from build123d import *

# Parameters (mm, degrees)
ESQUISSE1_W             = 180
ESQUISSE1_H             = 50
ESQUISSE1_R             = 3
BOSS_EXTRU_1_DEPTH      = 5
ESQUISSE2_W             = 75
ESQUISSE2_H             = 15
BOSS_EXTRU_2_DEPTH      = 75
ESQUISSE3_R             = 15
ENL_V_MAT_EXTRU_1_DEPTH = 15
ESQUISSE4_R             = 31
ENL_V_MAT_EXTRU_2_DEPTH = 10
CONG_1_R                = 20
CHANFREIN1_SIZE         = 15
CHANFREIN1_SIZE2        = 12.586494468
CONG_2_R                = 20
ESQUISSE5_W             = 10
ESQUISSE5_H             = 10
ENL_V_MAT_EXTRU_3_DEPTH = 5


with BuildPart() as part:
    # Esquisse1 → Boss.-Extru.1 (new body)
    with BuildSketch(Plane.XY):
        with Locations((5.796013405, 25)):
            Rectangle(ESQUISSE1_W, ESQUISSE1_H)
        with Locations((40.796013405, 6)):
            Circle(ESQUISSE1_R, mode=Mode.SUBTRACT)
        with Locations((-69.406004871, 22.939397164)):
            Circle(ESQUISSE1_R, mode=Mode.SUBTRACT)
        with Locations((-40.981469067, 6.77616521)):
            Circle(ESQUISSE1_R, mode=Mode.SUBTRACT)
        with Locations((-8.861542866, 12.901085106)):
            Circle(ESQUISSE1_R, mode=Mode.SUBTRACT)
        with Locations(Location((-29.203986595, 6, 0), (0, 0, 180))):
            Circle(ESQUISSE1_R, mode=Mode.SUBTRACT)
        with Locations(Location((80.99803168, 22.939397164, 0), (0, 0, 180))):
            Circle(ESQUISSE1_R, mode=Mode.SUBTRACT)
        with Locations(Location((52.573495876, 6.77616521, 0), (0, 0, 180))):
            Circle(ESQUISSE1_R, mode=Mode.SUBTRACT)
        with Locations(Location((20.453569676, 12.901085106, 0), (0, 0, 180))):
            Circle(ESQUISSE1_R, mode=Mode.SUBTRACT)
    extrude(amount=BOSS_EXTRU_1_DEPTH)

    # Esquisse2 → Boss.-Extru.2 (add)
    with BuildSketch(Plane.XY.offset(5)):
        with Locations((5.796013405, 42.5)):
            Rectangle(ESQUISSE2_W, ESQUISSE2_H)
    extrude(amount=BOSS_EXTRU_2_DEPTH)

    # Esquisse3 → Enlèv. mat.-Extru.1 (cut)
    with BuildSketch(Plane(origin=(0, 50, 0), x_dir=(1, 0, 0), z_dir=(0, 1, 0))):
        with Locations(Location((5.796013405, -42.5, 0), (0, 0, 270))):
            Circle(ESQUISSE3_R)
    extrude(amount=-ENL_V_MAT_EXTRU_1_DEPTH, mode=Mode.SUBTRACT)

    # Esquisse4 → Enlèv. mat.-Extru.2 (cut)
    with BuildSketch(Plane(origin=(0, 50, 0), x_dir=(1, 0, 0), z_dir=(0, 1, 0))):
        with Locations(Location((5.796013405, -42.5, 0), (0, 0, 270))):
            Circle(ESQUISSE4_R)
    extrude(amount=-ENL_V_MAT_EXTRU_2_DEPTH, mode=Mode.SUBTRACT)

    # Congé1
    cong_1_edges = [part.edges().sort_by_distance(p)[0] for p in [
        (43.296013405, 42.5, 80),
        (-31.703986595, 42.5, 80),
    ]]
    fillet(cong_1_edges, radius=CONG_1_R)

    # Chanfrein1
    chanfrein1_edges = [part.edges().sort_by_distance(p)[0] for p in [
        (5.796013405, 35, 5),
    ]]
    chanfrein1_side = [part.faces().sort_by_distance(p)[0] for p in [
        (5.796013405, 22.805952806, 5),
    ]]
    chamfer(chanfrein1_edges, length=CHANFREIN1_SIZE, length2=CHANFREIN1_SIZE2, reference=chanfrein1_side[0])

    # Congé2
    # the kernel refuses this fillet: 20 mm, written as the material it adds along each edge
    with BuildSketch(Plane(origin=(-31.703986595, -30, 5), x_dir=(0, 0, 1), z_dir=(0, 1, 0))) as cong_2_piece_1_section:
        with BuildLine():
            CenterArc((CONG_2_R, -CONG_2_R), CONG_2_R, 90, 90)
            Line((0, -CONG_2_R), (0, 0))
            Line((0, 0), (CONG_2_R, 0))
        make_face()
    cong_2_piece_1 = extrude(amount=80, mode=Mode.PRIVATE)
    cong_2_piece_1 = split(cong_2_piece_1, bisect_by=Plane(origin=(-37.472324852, 26.525505275, 10.475549069), z_dir=(0, 0.6427876096865406, -0.766044443118977)), keep=Keep.TOP, mode=Mode.PRIVATE)
    cong_2_piece_1 = split(cong_2_piece_1, bisect_by=Plane(origin=(-37.472324852, 35, 7.522714945), z_dir=(0, -1, 0)), keep=Keep.TOP, mode=Mode.PRIVATE)
    add(cong_2_piece_1)
    with BuildSketch(Plane(origin=(-31.703986595, -30, 5), x_dir=(0, 0, 1), z_dir=(0, 1, 0))) as cong_2_piece_2_section:
        with BuildLine():
            CenterArc((CONG_2_R, -CONG_2_R), CONG_2_R, 90, 90)
            Line((0, -CONG_2_R), (0, 0))
            Line((0, 0), (CONG_2_R, 0))
        make_face()
    cong_2_piece_2 = extrude(amount=80, mode=Mode.PRIVATE)
    cong_2_piece_2 = split(cong_2_piece_2, bisect_by=Plane(origin=(-31.680860217, 38.546515029, 20.562373921), z_dir=(0, -0.6427876096865406, 0.766044443118977)), keep=Keep.TOP, mode=Mode.PRIVATE)
    cong_2_piece_2 = split(cong_2_piece_2, bisect_by=Plane(origin=(-31.680860217, 35, 21.798113742), z_dir=(0, 1, 0)), keep=Keep.TOP, mode=Mode.PRIVATE)
    add(cong_2_piece_2)
    with BuildSketch(Plane(origin=(-31.703986595, -30, 5), x_dir=(0, 0, 1), z_dir=(0, 1, 0))) as cong_2_piece_3_section:
        with BuildLine():
            CenterArc((CONG_2_R, -CONG_2_R), CONG_2_R, 90, 90)
            Line((0, -CONG_2_R), (0, 0))
            Line((0, 0), (CONG_2_R, 0))
        make_face()
    cong_2_piece_3 = extrude(amount=80, mode=Mode.PRIVATE)
    cong_2_piece_3 = split(cong_2_piece_3, bisect_by=Plane(origin=(-36.294325359, 35.39038505, 17.914066419), z_dir=(0, 0.6427876096865406, -0.766044443118977)), keep=Keep.TOP, mode=Mode.PRIVATE)
    cong_2_piece_3 = split(cong_2_piece_3, bisect_by=Plane(origin=(-36.294325359, 35, 9.359564784), z_dir=(0, 1, 0)), keep=Keep.TOP, mode=Mode.PRIVATE)
    add(cong_2_piece_3)
    with BuildSketch(Plane(origin=(43.296013405, -30, 5), x_dir=(0, 0, 1), z_dir=(0, 1, 0))) as cong_2_piece_4_section:
        with BuildLine():
            CenterArc((CONG_2_R, CONG_2_R), CONG_2_R, 180, 90)
            Line((0, CONG_2_R), (0, 0))
            Line((0, 0), (CONG_2_R, 0))
        make_face()
    cong_2_piece_4 = extrude(amount=80, mode=Mode.PRIVATE)
    cong_2_piece_4 = split(cong_2_piece_4, bisect_by=Plane(origin=(49.064351662, 35, 7.522714945), z_dir=(0, -1, 0)), keep=Keep.TOP, mode=Mode.PRIVATE)
    cong_2_piece_4 = split(cong_2_piece_4, bisect_by=Plane(origin=(49.064351662, 26.525505275, 10.475549069), z_dir=(0, 0.6427876096865406, -0.766044443118977)), keep=Keep.TOP, mode=Mode.PRIVATE)
    add(cong_2_piece_4)
    with BuildSketch(Plane(origin=(43.296013405, -30, 5), x_dir=(0, 0, 1), z_dir=(0, 1, 0))) as cong_2_piece_5_section:
        with BuildLine():
            CenterArc((CONG_2_R, CONG_2_R), CONG_2_R, 180, 90)
            Line((0, CONG_2_R), (0, 0))
            Line((0, 0), (CONG_2_R, 0))
        make_face()
    cong_2_piece_5 = extrude(amount=80, mode=Mode.PRIVATE)
    cong_2_piece_5 = split(cong_2_piece_5, bisect_by=Plane(origin=(43.272887026, 35, 21.798113742), z_dir=(0, 1, 0)), keep=Keep.TOP, mode=Mode.PRIVATE)
    cong_2_piece_5 = split(cong_2_piece_5, bisect_by=Plane(origin=(43.272887026, 38.546515029, 20.562373921), z_dir=(0, -0.6427876096865406, 0.766044443118977)), keep=Keep.TOP, mode=Mode.PRIVATE)
    add(cong_2_piece_5)
    with BuildSketch(Plane(origin=(43.296013405, -30, 5), x_dir=(0, 0, 1), z_dir=(0, 1, 0))) as cong_2_piece_6_section:
        with BuildLine():
            CenterArc((CONG_2_R, CONG_2_R), CONG_2_R, 180, 90)
            Line((0, CONG_2_R), (0, 0))
            Line((0, 0), (CONG_2_R, 0))
        make_face()
    cong_2_piece_6 = extrude(amount=80, mode=Mode.PRIVATE)
    cong_2_piece_6 = split(cong_2_piece_6, bisect_by=Plane(origin=(47.886352168, 35, 9.359564784), z_dir=(0, 1, 0)), keep=Keep.TOP, mode=Mode.PRIVATE)
    cong_2_piece_6 = split(cong_2_piece_6, bisect_by=Plane(origin=(47.886352168, 35.39038505, 17.914066419), z_dir=(0, 0.6427876096865406, -0.766044443118977)), keep=Keep.TOP, mode=Mode.PRIVATE)
    add(cong_2_piece_6)

    # Esquisse5 → Enlèv. mat.-Extru.3 (cut)
    with BuildSketch(Plane.XY.offset(5)):
        with Locations((-79.203986595, 5)):
            Rectangle(ESQUISSE5_W, ESQUISSE5_H)
        with Locations((90.796013405, 5)):
            Rectangle(ESQUISSE5_W, ESQUISSE5_H)
    extrude(amount=-ENL_V_MAT_EXTRU_3_DEPTH, mode=Mode.SUBTRACT)


solid = part.part
Work out the finished part from the listing and answer in its coordinate system (mm). A direction names the side the tool comes from. Round coordinates to 2 decimals unless told otherwise and drop trailing zeros. Write each loop counter-clockwise with the first axis right and the second up, starting at its lowest first coordinate (ties: lowest second). Pieces come first, ordered by that corner, then holes. Notation, with made-up numbers: (77, 84.25) -> (126, 84.25) arc R22 cw to (126, 93.25) -> close; hole circle Ø3 at (-8.5, 55). An arc over 180 degrees is marked (long way). Write each question's results on one line, items separated by ' | '.
Item 1: Flat-ended cylindrical pins translate along their axes: P1, Ø2, axis at x = 46, z = 56, coming from the +Y side; P2, Ø8, axis at x = 52.57, y = 6.78, coming from the +Z side; P3, Ø2, axis at x = -11, y = 33, coming from the +Z side; P4, Ø8, axis at y = 28, z = 10.5, coming from the +X side. Find the tip coordinate at first contact, or state that the pin passes through.
Result set:
P1: through | P2: z = 5 | P3: z = 16.75 | P4: x = 55.7
Item 2: A cutting plane is placed at A-A, the plane z = 42.5. Determine the outline of the cut face in (x, y), plus the area to 3 significant figures.
Result set:
outline: (-31.7, 35) -> (-9.2, 35) -> (-9.2, 40) -> (-25.2, 40) -> (-25.2, 50) -> (-31.7, 50) -> close; (20.8, 35) -> (43.3, 35) -> (43.3, 50) -> (36.8, 50) -> (36.8, 40) -> (20.8, 40) -> close | area: 355 mm^2
Item 3: Which of the six approach directions +Z, -Z, +X, -X, +Y, -Y give full straight-line access (tool end or side, diameter ignored) to faces 4 (the face through (15, 35, 55)), 5 (the face through (43.296, 42, 42)), 6 (the face through (43.567, 4.851, 2.465)), 7 (the face through (13, 40, 56)), 8 (the face through (-74.204, 5, 3))?
Result set:
face 4: +Z, +X, -X, -Y | face 5: +Z, +X, +Y, -Y | face 6: +Z, -Z | face 7: +Y | face 8: +Z, -Z, -X, -Y
Item 4: Find the intervals of material crossed by line 1 along Z through (x, y) = (24, 19); line 2 along X through (y, z) = (36.45, 42.5); line 3 along Y through (x, z) = (-19, 47), in increasing order. Write a range as [from, to].
Result set:
line 1: [0, 5] | line 2: [-31.7, -9.2], [20.8, 43.3] | line 3: [35, 40]
Item 5: A cutting plane is placed at B-B, the plane x = -29. Determine the outline of the cut face in (y, z), plus the area to 3 significant figures.
Result set:
outline: (0, 0) -> (3.01, 0) -> (3.01, 5) -> (0, 5) -> close; (8.99, 0) -> (50, 0) -> (50, 70.04) -> (35, 70.04) -> (35, 17.59) -> (20, 5) -> (8.99, 5) -> close | area: 1,290 mm^2
Item 6: The mould has two halves that part along X. Classify faces 1 (the face through (4.5, 19.8, 5)), 2 (the face through (-66.545, 23.841, 2.465)), 3 (the face through (37.28, 42.6, 74.3)): +X half, -X half, draft (parallel to the pull), parting line (faces both ways), or undercut.
Result set:
face 1: draft | face 2: undercut | face 3: +X half
Item 7: A cutting plane is placed at C-C, the plane y = 29. Determine the outline of the cut face in (x, z), plus the area to 3 significant figures.
Result set:
outline: (-84.2, 0) -> (95.8, 0) -> (95.8, 5) -> (63.3, 5) arc R20 cw to (47.64, 12.55) -> (-36.05, 12.55) arc R20 cw to (-51.7, 5) -> (-84.2, 5) -> close | area: 1,600 mm^2
Item 8: A cutting plane is placed at D-D, the plane z = 33.5. Determine the outline of the cut face in (x, y), plus the area to 3 significant figures.
Result set:
outline: (-31.7, 35) -> (-6.2, 35) -> (-6.2, 40) -> (-23.87, 40) -> (-23.87, 50) -> (-31.7, 50) -> close; (17.8, 35) -> (43.3, 35) -> (43.3, 50) -> (35.46, 50) -> (35.46, 40) -> (17.8, 40) -> close | area: 412 mm^2
